```python
from build123d import *

# Parameters (mm, degrees)
F1_W = 100
F1_H = 100
F2_W = 40
F2_H = 15
F4_T = -3


with BuildPart() as f3:
    # F1 (on offset) → F3 section 0
    with BuildSketch(Plane.XY.offset(100)):
        with Locations((50, -50)):
            Rectangle(F1_W, F1_H)
    # F2 (on Top) → F3 section 1
    with BuildSketch(Plane.XY):
        with Locations((55, -50.5)):
            Rectangle(F2_W, F2_H)
    loft()

    # F4
    f4_openings = [f3.faces().sort_by_distance(p)[0] for p in [
        (50, -50, 100),
        (55, -50.5, 0),
    ]]
    offset(amount=F4_T, openings=f4_openings, kind=Kind.INTERSECTION)


solid = f3.part
```
Geometry check sheet. Reference: the model listing, model coordinates, mm. Give positions to 0.01 mm unless a question says otherwise; leave off trailing zeros. Write item = value, one per line.
(1) Material ranges on line 1 (X direction, y = -18.5, z = 68.5) (3 decimals); line 2 (Y direction, x = 49.5, z = 4); line 3 (Y direction, x = 62, z = 87), recorded low to high. Write a range as [from, to].
Answer below:
line_1 = [11.025, 14.203], [89.033, 92.125]
line_2 = [-59.68, -56.43], [-44.55, -41.28]
line_3 = [-94.54, -91.29], [-8.86, -5.59]
(2) Gauge pin test, flat ends, axial feed: pin 1 Ø3 at (x, z) = (53.5, 69.5) entering from +Y; pin 2 Ø2 at (x, z) = (21.5, 64.5) entering from +Y (3 decimals); pin 3 Ø2 at (y, z) = (-59, 48) entering from +X. Record the tip position at first contact, or that the pin passes through.
Answer below:
pin_1 = -12.47
pin_2 = -14.835
pin_3 = 87.25
(3) Release check for a two-part mould opening along Y. For faces 1 (the face through (87.062, -50.977, 60.618)), 2 (the face through (53, -2, 100)) record: released by +Y, released by -Y, zero draft, split by the parting line, or undercut.
Answer below:
face_1 = undercut
face_2 = zero draft
